The listing builds one solid part. Answer for the finished solid, in the listing's coordinates (mm). Face numbers are marked on the shaded views. A direction names the side the tool comes from. Coordinates: 2 decimals unless noted, no trailing zeros. Loops run counter-clockwise (first coordinate to the right, second up) from the corner with the lowest first, then second, coordinate; pieces in that order, holes last. Notation, with made-up numbers: (-17, -18) -> (15, -18) arc R36 ccw to (15, 16) -> close; hole circle Ø1 at (89, 60). An arc over 180 degrees is marked (long way). Answer in a Markdown table with one row per item.
```python
from build123d import *

# Parameters (mm, degrees)
F1_DEPTH = 55.88
F3_DEPTH = 54.38
F4_R     = 2.1556257218
F4_R_2   = 2.2
F5_DEPTH = 1.501


with BuildPart() as f1:
    # F0 (on Top) → F1 (new body)
    with BuildSketch(Plane.XY):
        with BuildLine():
            Line((26.67, 35.56), (-26.67, 35.56))
            ThreePointArc((-26.67, 35.56), (-48.2226146906, 26.6326146906), (-57.15, 5.08))
            Line((-57.15, 5.08), (-57.15, -5.08))
            ThreePointArc((-57.15, -5.08), (-48.2226146906, -26.6326146906), (-26.67, -35.56))
            Line((-26.67, -35.56), (26.67, -35.56))
            ThreePointArc((26.67, -35.56), (48.2226146906, -26.6326146906), (57.15, -5.08))
            Line((57.15, -5.08), (57.15, 5.08))
            ThreePointArc((57.15, 5.08), (48.2226146906, 26.6326146906), (26.67, 35.56))
        make_face()
    extrude(amount=F1_DEPTH)

    # F2 (on face) → F3 (cut, through all)
    with BuildSketch(Plane.XY.offset(55.88)):
        with BuildLine():
            ThreePointArc((48.9134000813, 19.1371286276), (25.6668993073, 30.4909660232), (0, 33.734375))
            ThreePointArc((0, 33.734375), (-25.6668993073, 30.4909660232), (-48.9134000813, 19.1371286276))
            ThreePointArc((-48.9134000813, 19.1371286276), (-52.0514727222, 15.5164140041), (-53.18125, 10.8601625518))
            Line((-53.18125, 10.8601625518), (-53.18125, 0))
            Line((-53.18125, 0), (-53.18125, -10.8601625518))
            ThreePointArc((-53.18125, -10.8601625518), (-52.0514727222, -15.5164140041), (-48.9134000813, -19.1371286276))
            ThreePointArc((-48.9134000813, -19.1371286276), (-25.6668993073, -30.4909660232), (0, -33.734375))
            ThreePointArc((0, -33.734375), (25.6668993073, -30.4909660232), (48.9134000813, -19.1371286276))
            ThreePointArc((48.9134000813, -19.1371286276), (52.0514727222, -15.5164140041), (53.18125, -10.8601625518))
            Line((53.18125, -10.8601625518), (53.18125, 0))
            Line((53.18125, 0), (53.18125, 10.8601625518))
            ThreePointArc((53.18125, 10.8601625518), (52.0514727222, 15.5164140041), (48.9134000813, 19.1371286276))
        make_face()
    extrude(amount=-F3_DEPTH, mode=Mode.SUBTRACT)

    # F4 (on face) → F5 (cut, through all)
    with BuildSketch(Plane.XY.offset(1.5)):
        with Locations((-25.4, 0)):
            Circle(F4_R)
        with Locations((25.4, 0)):
            Circle(F4_R_2)
    extrude(amount=-F5_DEPTH, mode=Mode.SUBTRACT)


solid = f1.part
```
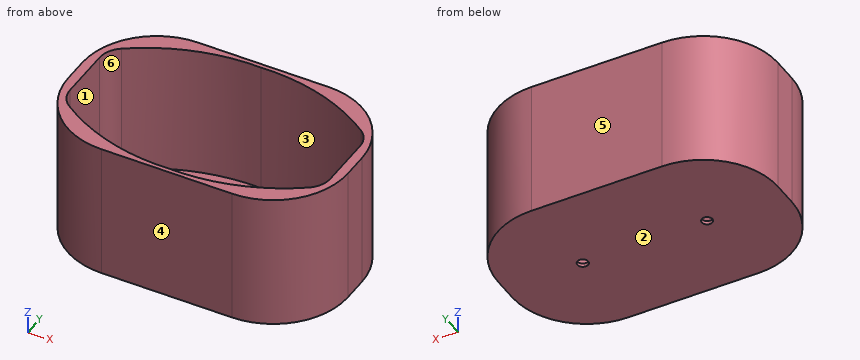
Item 1: Determine the mould class of the marked faces 3, 4, 5 and 6 for opening direction Y: +Y half, -Y half, draft (parallel to the pull), parting line (faces both ways), or undercut.
Findings below:
| item | result |
|---|---|
| face 3 | undercut |
| face 4 | -Y half |
| face 5 | +Y half |
| face 6 | undercut |
Item 2: A cutting plane is placed at A-A, the plane y = 0. Determine the outline of the cut face in (x, z), plus the area to 3 significant figures.
Findings below:
| item | result |
|---|---|
| outline | (-57.15, 0) -> (-27.56, 0) -> (-27.56, 1.5) -> (-53.18, 1.5) -> (-53.18, 55.88) -> (-57.15, 55.88) -> close; (-23.24, 0) -> (23.2, 0) -> (23.2, 1.5) -> (-23.24, 1.5) -> close; (27.6, 0) -> (57.15, 0) -> (57.15, 55.88) -> (53.18, 55.88) -> (53.18, 1.5) -> (27.6, 1.5) -> close |
| area | 590 mm2 |
Item 3: A tool of negligible diameter and unlimited length cuts with its end or side. For the marked faces 1 and 2, from which of +Z, -Z, +X, -X, +Y, -Y can it reach the whole face along a straight path? Write none if from no direction.
Findings below:
| item | result |
|---|---|
| face 1 | +Z |
| face 2 | -Z, +X, -X, +Y, -Y |
Item 4: Flat-ended cylindrical pins translate along their axes: pin 1 Ø2 at (y, z) = (20, 20.5) entering from +X; pin 2 Ø2.5 at (x, y) = (25.4, 0) entering from +Z; pin 3 Ø4 at (x, y) = (6.5, 7.5) entering from +Z; pin 4 Ø10 at (y, z) = (-22, 36.5) entering from +X. Find the tip coordinate at first contact, or state that the pin passes through.
Findings below:
| item | result |
|---|---|
| pin 1 | stops at x = 53.79 |
| pin 2 | passes through |
| pin 3 | stops at z = 1.5 |
| pin 4 | stops at x = 54.72 |
Item 5: A cutting plane is placed at D-D, the plane x = 10. Determine the outline of the cut face in (y, z).
Findings below:
| item | result |
|---|---|
| outline | (-35.56, 0) -> (35.56, 0) -> (35.56, 55.88) -> (33.49, 55.88) -> (33.49, 1.5) -> (-33.49, 1.5) -> (-33.49, 55.88) -> (-35.56, 55.88) -> close |
Item 6: A cutting plane is placed at C-C, the plane z = 12. Determine the outline of the cut face in (x, y).
Findings below:
| item | result |
|---|---|
| outline | (-57.15, -5.08) arc R30.48 ccw to (-26.67, -35.56) -> (26.67, -35.56) arc R30.48 ccw to (57.15, -5.08) -> (57.15, 5.08) arc R30.48 ccw to (26.67, 35.56) -> (-26.67, 35.56) arc R30.48 ccw to (-57.15, 5.08) -> close; hole (-53.18, -10.86) arc R10.16 ccw to (-48.91, -19.14) arc R79.08 ccw to (0, -33.73) arc R79.08 ccw to (48.91, -19.14) arc R10.16 ccw to (53.18, -10.86) -> (53.18, 10.86) arc R10.16 ccw to (48.91, 19.14) arc R79.08 ccw to (0, 33.73) arc R79.08 ccw to (-48.91, 19.14) arc R10.16 ccw to (-53.18, 10.86) -> close |
Item 7: Find the intervals of material crossed by probe 1 along X at (y, z) = (-5, 41.5); probe 2 along Y at (x, z) = (25.4, 1.05); probe 3 along Z at (x, y) = (11, -14), in increasing order.
Findings below:
| item | result |
|---|---|
| probe 1 | x = -57.15 to -53.18, 53.18 to 57.15 |
| probe 2 | y = -35.56 to -2.2, 2.2 to 35.56 |
| probe 3 | z = 0 to 1.5 |
Item 8: A cutting plane is placed at B-B, the plane x = 25.4. Determine the outline of the cut face in (y, z), plus the area to 3 significant figures.
Findings below:
| item | result |
|---|---|
| outline | (-35.56, 0) -> (-2.2, 0) -> (-2.2, 1.5) -> (-30.57, 1.5) -> (-30.57, 55.88) -> (-35.56, 55.88) -> close; (2.2, 0) -> (35.56, 0) -> (35.56, 55.88) -> (30.57, 55.88) -> (30.57, 1.5) -> (2.2, 1.5) -> close |
| area | 643 mm2 |
